```python
from build123d import *

# Parameters (mm, degrees)
BOSS_EXTRUDE1_DEPTH = 76.2


with BuildPart() as part:
    # Sketch2 → Boss-Extrude1 (new body, symmetric)
    with BuildSketch(Plane.XY):
        with BuildLine():
            Line((0, 0), (0, 50.8))
            Line((0, 50.8), (6.35, 50.8))
            Line((6.35, 50.8), (6.35, 12.7))
            ThreePointArc((6.35, 12.7), (8.209871939, 8.209871939), (12.7, 6.35))
            Line((12.7, 6.35), (50.8, 6.35))
            Line((50.8, 6.35), (50.8, 0))
            Line((50.8, 0), (0, 0))
        make_face()
    extrude(amount=BOSS_EXTRUDE1_DEPTH, both=True)


solid = part.part
```
Check sheet for the modelled part. Datum: model origin and axes. Units: mm. A direction names the side the tool comes from. Coordinates: 2 decimals unless noted, no trailing zeros. Write each loop counter-clockwise with the first axis right and the second up, starting at its lowest first coordinate (ties: lowest second). Pieces come first, ordered by that corner, then holes. Notation, with made-up numbers: (-8, 18) -> (50, 18) arc R16 cw to (50, 25) -> close; hole circle Ø8 at (27, 52.5). An arc over 180 degrees is marked (long way). Use a Markdown table: item, result.
1. Sectioned sample at A-A (z = -56.5). Enter the section's corners in (x, y), plus the area to 3 significant figures.
Reported:
| item | result |
|---|---|
| outline | (0, 0) -> (50.8, 0) -> (50.8, 6.35) -> (12.7, 6.35) arc R6.35 cw to (6.35, 12.7) -> (6.35, 50.8) -> (0, 50.8) -> close |
| area | 613 mm2 |
2. Sectioned sample at B-B (y = 17.5). Enter the section's corners in (x, z), plus the area to 3 significant figures.
Reported:
| item | result |
|---|---|
| outline | (0, -76.2) -> (6.35, -76.2) -> (6.35, 76.2) -> (0, 76.2) -> close |
| area | 968 mm2 |
3. Go/stop test with flat-tipped pins: pin 1 Ø6 at (y, z) = (22, -34) entering from +X; pin 2 Ø19 at (x, z) = (36, -6) entering from +Y. Record where each tip stops, or that it passes through.
Reported:
| item | result |
|---|---|
| pin 1 | stops at x = 6.35 |
| pin 2 | stops at y = 6.35 |
4. Scan lines: line 1 along Y through (x, z) = (46.5, 13.5); line 2 along Y through (x, z) = (9, -38). Record each from-to range of solid material in increasing order.
Reported:
| item | result |
|---|---|
| line 1 | y = 0 to 6.35 |
| line 2 | y = 0 to 7.54 |
5. Tool access check on faces 1 (the flat face through (31, 6.35, 1)), 2 (the flat face through (0, 25, 1)). Record the directions out of +Z, -Z, +X, -X, +Y, -Y that give a thin tool (end or side, any length) a straight path to the whole face; none if there is none.
Reported:
| item | result |
|---|---|
| face 1 | +Z, -Z, +X, +Y |
| face 2 | +Z, -Z, -X, +Y, -Y |
